```python
from build123d import *

# Parameters (mm, degrees)
F1_DEPTH = 101.6
F2_R     = 1.98374
F3_R     = 3.69316
F4_W     = 9.5329248
F4_H     = 24
F4_R     = 1.35255
F4_R_2   = 1.8288
F5_DEPTH = 257
F6_R     = 1.8288
F7_DEPTH = 136.06526


# Not quite as in the source:
# - an extrude ends at something that could not be found from the text; its depth is read off the source's solid


with BuildPart() as f1:
    # F0 (on Top) → F1 (new body)
    with BuildSketch(Plane.XY):
        Polygon((0, 29.2656006), (0, 0), (-132.64642, 0), (-132.64642, 29.2656006), (-134.35584, 29.2656006), (-134.35584, -1.70942), (1.70942, -1.70942), (1.70942, 29.2656006), align=None)
    extrude(amount=F1_DEPTH)

    # F2
    f2_edges = [f1.edges().sort_by_distance(p)[0] for p in [
        (0, 0, 50.8),
        (-132.64642, 0, 50.8),
    ]]
    fillet(f2_edges, radius=F2_R)

    # F3
    f3_edges = [f1.edges().sort_by_distance(p)[0] for p in [
        (-134.35584, -1.70942, 50.8),
        (1.70942, -1.70942, 50.8),
    ]]
    fillet(f3_edges, radius=F3_R)

    # F4 (on face) → F5 (cut, through all)
    with BuildSketch(Plane.XZ.offset(1.70942)):
        with Locations((-9.48374, 15.175)):
            Rectangle(F4_W, F4_H)
        with Locations((-123.16268, 15.175)):
            Rectangle(F4_W, F4_H)
        with Locations((-123.16268, 86.425)):
            Rectangle(F4_W, F4_H)
        with Locations((-9.48374, 86.425)):
            Rectangle(F4_W, F4_H)
        with Locations((-24.6456604, 7.14375)):
            Circle(F4_R)
        with Locations((-108.0007596, 7.14375)):
            Circle(F4_R)
        with Locations((-108.0007596, 94.45625)):
            Circle(F4_R)
        with Locations((-24.6456604, 94.45625)):
            Circle(F4_R)
        with Locations((-59.97321, 3.175)):
            Circle(F4_R_2)
        with Locations((-72.67321, 3.175)):
            Circle(F4_R_2)
        with Locations((-59.97321, 98.425)):
            Circle(F4_R_2)
        with Locations((-72.67321, 98.425)):
            Circle(F4_R_2)
    extrude(amount=-F5_DEPTH, mode=Mode.SUBTRACT)

    # F6 (on face) → F7 (cut, through all)
    with BuildSketch(Plane(origin=(-134.35584, 0, 0), x_dir=(0, -1, 0), z_dir=(-1, 0, 0))):
        with Locations((-26.0906006, 3.175)):
            Circle(F6_R)
        with Locations((-13.3906006, 3.175)):
            Circle(F6_R)
        with Locations((-13.3906006, 98.425)):
            Circle(F6_R)
        with Locations((-26.0906006, 98.425)):
            Circle(F6_R)
    extrude(amount=-F7_DEPTH, mode=Mode.SUBTRACT)


solid = f1.part
```
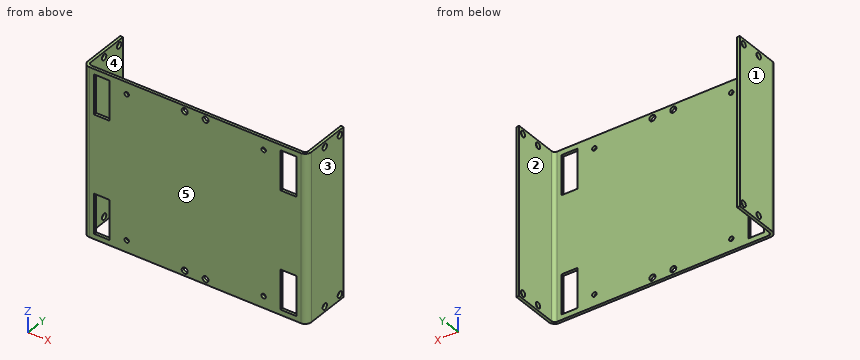
Build history of the part. All positions in model axes, mm. Face numbers are marked on the shaded views. A direction names the side the tool comes from. Give positions to 0.01 mm unless a question says otherwise; leave off trailing zeros. Loops run counter-clockwise (first coordinate to the right, second up) from the corner with the lowest first, then second, coordinate; pieces in that order, holes last. Notation, with made-up numbers: (-35, 14) -> (-21, 14) arc R30 cw to (-21, 48) -> close; hole circle Ø1 at (36.5, 62). An arc over 180 degrees is marked (long way). One line per question, with ' | ' between items.
Q1. Pull direction X, two halves, no side cores. Call the marked faces 3, 4 and 5: pulls with the +X half, pulls with the -X half, needs draft (parallel to the pull), parting line crosses it, or undercut.
Filled sheet:
face 3: pulls with the +X half | face 4: undercut | face 5: needs draft
Q2. Cut at C-C, the plane x = -9. Write the cut outline in (y, z) (3 decimals).
Filled sheet:
outline: (-1.709, 0) -> (0, 0) -> (0, 3.175) -> (-1.709, 3.175) -> close; (-1.709, 27.175) -> (0, 27.175) -> (0, 74.425) -> (-1.709, 74.425) -> close; (-1.709, 98.425) -> (0, 98.425) -> (0, 101.6) -> (-1.709, 101.6) -> close
Q3. Cut at A-A, the plane z = 85.5. Write the cut outline in (x, y), plus the area to 3 significant figures.
Filled sheet:
outline: (-134.36, 1.98) arc R3.69 ccw to (-130.66, -1.71) -> (-127.93, -1.71) -> (-127.93, 0) -> (-130.66, 0) arc R1.98 cw to (-132.65, 1.98) -> (-132.65, 29.27) -> (-134.36, 29.27) -> close; (-118.4, -1.71) -> (-14.25, -1.71) -> (-14.25, 0) -> (-118.4, 0) -> close; (-4.72, -1.71) -> (-1.98, -1.71) arc R3.69 ccw to (1.71, 1.98) -> (1.71, 29.27) -> (0, 29.27) -> (0, 1.98) arc R1.98 cw to (-1.98, 0) -> (-4.72, 0) -> close | area: 296 mm²
Q4. Tool access for the marked faces 1 and 2: list every direction of +Z, -Z, +X, -X, +Y, -Y with a clear straight run to the whole face (end or side of a thin tool).
Filled sheet:
face 1: +Z, -Z, -X, +Y, -Y | face 2: +Z, -Z, +Y
Q5. Drop flat-ended pins along their axis: pin 1 (12 mm diameter, centred on x = -106, y = 7.5, fed in from +Z); pin 2 (0.9 mm diameter, centred on y = -1, z = 82, fed in from +X); pin 3 (3 mm diameter, centred on x = -92.5, z = 60.5, fed in from +Y); pin 4 (1.4 mm diameter, centred on y = -1, z = 20, fed in from +X). Give the stop position or say it passes through.
Filled sheet:
pin 1: passes through | pin 2: stops at x = 0.7 | pin 3: stops at y = 0 | pin 4: stops at x = 0.92
Q6. Drill centre lines: line 1 along X through (y, z) = (4, 24.5); line 2 along Y through (x, z) = (-71, 54.5); line 3 along X through (y, z) = (1.5, 71). Where is each one in solid material? Low to high. Write a range as [from, to].
Filled sheet:
line 1: x = [-134.36, -132.65], [0, 1.71] | line 2: y = [-1.71, 0] | line 3: x = [-134.32, -132.59], [-0.06, 1.68]
Q7. Cut at D-D, the plane z = 70.5. Write the cut outline in (x, y), plus the area to 3 significant figures.
Filled sheet:
outline: (-134.36, 1.98) arc R3.69 ccw to (-130.66, -1.71) -> (-1.98, -1.71) arc R3.69 ccw to (1.71, 1.98) -> (1.71, 29.27) -> (0, 29.27) -> (0, 1.98) arc R1.98 cw to (-1.98, 0) -> (-130.66, 0) arc R1.98 cw to (-132.65, 1.98) -> (-132.65, 29.27) -> (-134.36, 29.27) -> close | area: 328 mm²
Q8. Cut at B-B, the plane y = 19. Write the cut outline in (x, z), plus the area to 3 significant figures.
Filled sheet:
outline: (-134.36, 0) -> (-132.65, 0) -> (-132.65, 101.6) -> (-134.36, 101.6) -> close; (0, 0) -> (1.71, 0) -> (1.71, 101.6) -> (0, 101.6) -> close | area: 347 mm²
